Check sheet for the modelled part. Datum: model origin and axes. Units: mm. Face numbers are marked on the shaded views. A direction names the side the tool comes from. Give positions to 0.01 mm unless a question says otherwise; leave off trailing zeros. Write each loop counter-clockwise with the first axis right and the second up, starting at its lowest first coordinate (ties: lowest second). Pieces come first, ordered by that corner, then holes.
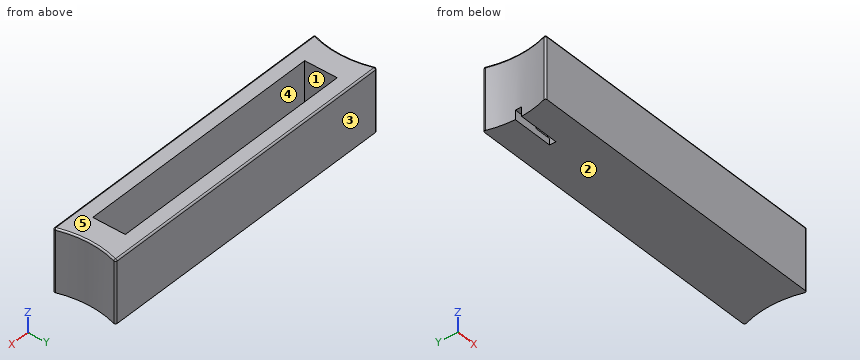
from build123d import *

# Parameters (mm, degrees)
CYLINDER_R        = 30
CYLINDER_DEPTH    = 20
CYLINDER001_R     = 30
CYLINDER001_DEPTH = 20
BOX003_W          = 5.2
BOX003_H          = 10.4
BOX003_DEPTH      = 1
BOX002_W          = 15
BOX002_H          = 2
BOX002_DEPTH      = 3
BOX001_W          = 80.4
BOX001_H          = 10.4
BOX001_DEPTH      = 20
BOX_W             = 100
BOX_H             = 20
BOX_DEPTH         = 20
FILLET_R          = 0.5
FILLET001_R       = 0.5


with BuildPart() as cylinder:
    # Cylinder → Cylinder (new body)
    with BuildSketch(Plane(origin=(-28, 10, 0), x_dir=(1, 0, 0), z_dir=(0, 0, 1))):
        Circle(CYLINDER_R)
    extrude(amount=CYLINDER_DEPTH)


with BuildPart() as cylinder001:
    # Cylinder001 → Cylinder001 (new body)
    with BuildSketch(Plane(origin=(128, 10, 0), x_dir=(1, 0, 0), z_dir=(0, 0, 1))):
        Circle(CYLINDER001_R)
    extrude(amount=CYLINDER001_DEPTH)


with BuildPart() as cube003:
    # Box003 → Box003 (new body)
    with BuildSketch(Plane(origin=(9.8, 4.8, 2), x_dir=(1, 0, 0), z_dir=(0, 0, 1))):
        with Locations((2.6, 5.2)):
            Rectangle(BOX003_W, BOX003_H)
    extrude(amount=BOX003_DEPTH)


with BuildPart() as cube002:
    # Box002 → Box002 (new body)
    with BuildSketch(Plane(origin=(0, 9, 0), x_dir=(1, 0, 0), z_dir=(0, 0, 1))):
        with Locations((7.5, 1)):
            Rectangle(BOX002_W, BOX002_H)
    extrude(amount=BOX002_DEPTH)


with BuildPart() as cube001:
    # Box001 → Box001 (new body)
    with BuildSketch(Plane(origin=(9.8, 4.8, 3), x_dir=(1, 0, 0), z_dir=(0, 0, 1))):
        with Locations((40.2, 5.2)):
            Rectangle(BOX001_W, BOX001_H)
    extrude(amount=BOX001_DEPTH)


with BuildPart() as fillet001:
    # Box → Box (new body)
    with BuildSketch(Plane.XY):
        with Locations((50, 10)):
            Rectangle(BOX_W, BOX_H)
    extrude(amount=BOX_DEPTH)

    # Cut: cut Cube001
    add(cube001.part, mode=Mode.SUBTRACT)

    # Cut001: cut Cube002
    add(cube002.part, mode=Mode.SUBTRACT)

    # Cut002: cut Cube003
    add(cube003.part, mode=Mode.SUBTRACT)

    # Cut003: cut Cylinder001
    add(cylinder001.part, mode=Mode.SUBTRACT)

    # Cut004: cut Cylinder
    add(cylinder.part, mode=Mode.SUBTRACT)

    # Fillet
    fillet_edges = [fillet001.edges().sort_by_distance(p)[0] for p in [
        (99.715729, 20, 10),
        (0.284271, 20, 10),
        (99.715729, 0, 10),
        (0.284271, 0, 10),
    ]]
    fillet(fillet_edges, radius=FILLET_R)

    # Fillet001
    fillet001_edges = [fillet001.edges().sort_by_distance(p)[0] for p in [
        (50, 20, 20),
        (0.577865, 19.793369, 20),
        (99.422135, 19.793369, 20),
        (1.624557, 14.731343, 20),
        (98, 10, 20),
        (1.624557, 5.268657, 20),
        (99.422135, 0.206631, 20),
        (0.577865, 0.206631, 20),
        (50, 0, 20),
    ]]
    fillet(fillet001_edges, radius=FILLET001_R)


solid = fillet001.part
1) Sectioned sample at B-B on z = 17. Record the boundary of the cut face in (x, y).
2) Gauge pin test, flat ends, axial feed: pin 1 (2 mm diameter, centred on y = 12, z = 11.5, fed in from -X); pin 2 (5 mm diameter, centred on y = 7.5, z = 12, fed in from +X); pin 3 (1 mm diameter, centred on y = 3, z = 4, fed in from -X). Record the tip position at first contact, or that the pin passes through.
3) Scan lines: L1, parallel to Y at x = 83.5, z = 18.5; L2, parallel to X at y = 9.5, z = 4.5; L3, parallel to Z at x = 55, y = 5.5. Record each from-to range of solid material in increasing order.
4) Sectioned sample at A-A on y = 10. Record the boundary of the cut face in (x, z).
5) Access from +Z, -Z, +X, -X, +Y, -Y to the whole of each face (thin tool, end or side, straight path). Record for the marked faces 1 and 2.
6) Draft check along Y on the marked faces 3, 4 and 5. Enter one of: +Y half, -Y half, draft (parallel to the pull), parting line (faces both ways), or undercut.
7) Sectioned sample at C-C on x = 37. Record the boundary of the cut face in (y, z), then the cut area to 3 significant figures.
Answers below:
1. outline: (0.51, 0.66) arc R0.5 ccw to (0.98, 0) - (99.02, 0) arc R0.5 ccw to (99.49, 0.66) arc R30 cw to (99.49, 19.34) arc R0.5 ccw to (99.02, 20) - (0.98, 20) arc R0.5 ccw to (0.51, 19.34) arc R30 cw to start; hole (9.8, 4.8) - (90.2, 4.8) - (90.2, 15.2) - (9.8, 15.2) - close
2. pin 1: stops at x = 1.85
2. pin 2: stops at x = 98.42
2. pin 3: stops at x = 1.05
3. L1: y = 0 to 4.8, 15.2 to 20
3. L2: x = 2 to 9.8, 90.2 to 98
3. L3: z = 0 to 3
4. outline: (2, 3) - (9.8, 3) - (9.8, 20) - (2.5, 20) arc R0.5 ccw to (2, 19.5) - close; (15, 0) - (98, 0) - (98, 19.5) arc R0.5 ccw to (97.5, 20) - (90.2, 20) - (90.2, 3) - (15, 3) - close
5. face 1: +Z
5. face 2: -Z, +X, -X, +Y, -Y
6. face 3: +Y half
6. face 4: undercut
6. face 5: draft
7. outline: (0, 0) - (20, 0) - (20, 19.5) arc R0.5 ccw to (19.5, 20) - (15.2, 20) - (15.2, 3) - (4.8, 3) - (4.8, 20) - (0.5, 20) arc R0.5 ccw to (0, 19.5) - close
7. area: 223 mm2
